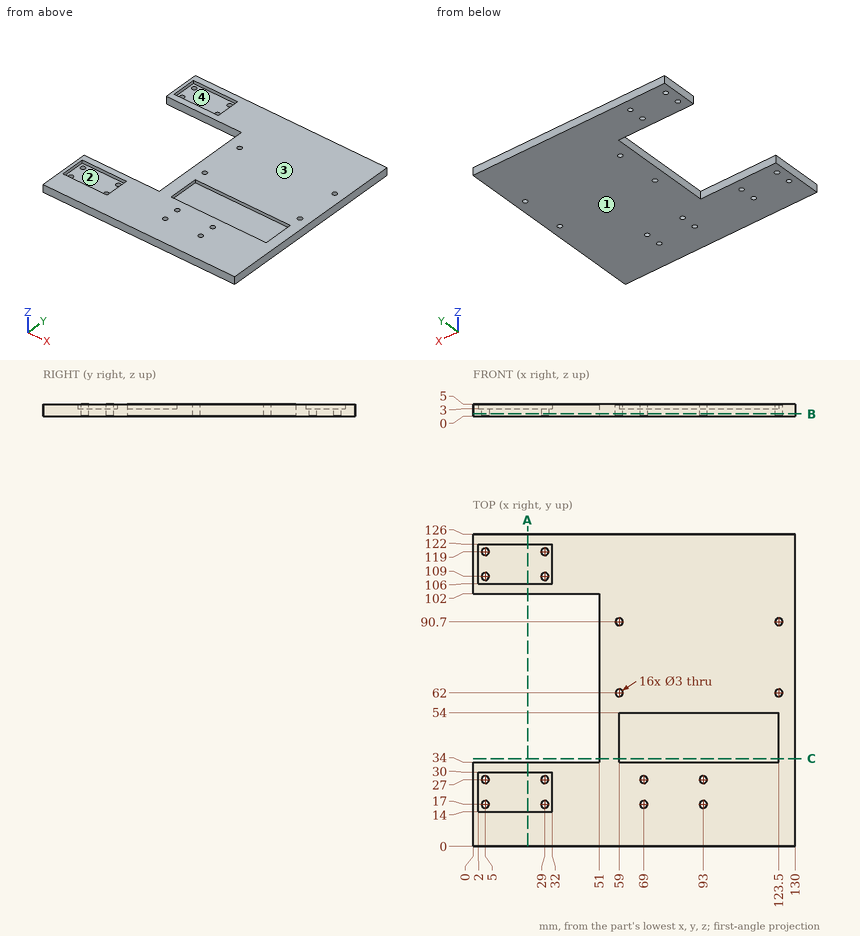
Study the drawing (mm; zero at the part's minimum x, y, z) and answer. A direction names the side the tool comes from. Give positions to 0.01 mm unless a question says otherwise; leave off trailing zeros. Order: outer loops, then holes, each group sorted by start corner. A loop starts at its lowest first (then second) coordinate and runs counter-clockwise, first axis right, second up. Notation, with made-up numbers: M 84,52.25 L 104,52.25 A25 ccw 104,75.25 Z; hole C -6.75,86 d5. An arc over 180 degrees is marked long. Put each result on its own line as item: value. Start each with the question number.
Item 1: The part is cut by section B-B, the plane z = 1. State how many separate pieces and enclosed holes the cut face has, and give its area (3 significant figures).
Item 2: Which of the six approach directions +Z, -Z, +X, -X, +Y, -Y give full straight-line access (tool end or side, diameter ignored) to the marked faces 3 and 4?
Item 3: For a pull along X with two mould halves and no side action, classify the marked faces 1 and 2 as +X half, -X half, draft (parallel to the pull), parting line (faces both ways), or undercut.
Item 4: Flat-ended cylindrical pins translate along their axes: P1, Ø4, axis at x = 69, y = 17, coming from the +Z side; P2, Ø5, axis at x = 5, y = 17, coming from the +Z side; P3, Ø2.5, axis at x = 93, y = 27, coming from the -Z side; P4, Ø2, axis at y = 49, z = 4.5, coming from the -X side. Find the tip coordinate at first contact, or state that the pin passes through.
Item 5: Find the intervals of material crossed by line 1 along Y through (x, z) = (93, 2.1); line 2 along X through (y, z) = (27, 1.9); line 3 along Y through (x, z) = (29, 1.1), in increasing order.
Item 6: The part is cut by section C-C, the plane y = 35.5. Determine the outline of the cut face in (x, z), and give its area (3 significant figures).
Item 7: The part is cut by section A-A, the plane x = 22. Determine the outline of the cut face in (y, z).
Answer key:
1. separate pieces: 1
1. enclosed holes: 16
1. area: 12,800 mm²
2. face 3: +Z, +X, -X, +Y, -Y
2. face 4: +Z
3. face 1: draft
3. face 2: undercut
4. P1: stops at z = 5
4. P2: stops at z = 3
4. P3: passes through
4. P4: stops at x = 51
5. line 1: y = 0 to 15.5, 18.5 to 25.5, 28.5 to 126
5. line 2: x = 0 to 3.5, 6.5 to 27.5, 30.5 to 67.5, 70.5 to 91.5, 94.5 to 130
5. line 3: y = 0 to 15.5, 18.5 to 25.5, 28.5 to 34, 102 to 107.5, 110.5 to 117.5, 120.5 to 126
6. outline: M 51,0 L 130,0 L 130,5 L 123.5,5 L 123.5,3 L 59,3 L 59,5 L 51,5 Z
6. area: 266 mm²
7. outline: M 0,0 L 34,0 L 34,5 L 30,5 L 30,3 L 14,3 L 14,5 L 0,5 Z; M 102,0 L 126,0 L 126,5 L 122,5 L 122,3 L 106,3 L 106,5 L 102,5 Z
